Geometry: final body of the model. Coordinates: model frame, mm. A direction names the side the tool comes from. Give positions to 0.01 mm unless a question says otherwise; leave off trailing zeros. Write each loop counter-clockwise with the first axis right and the second up, starting at its lowest first coordinate (ties: lowest second). Pieces come first, ordered by that corner, then holes. Notation, with made-up numbers: M 57,0 L 66,0 A35 ccw 66,37 Z; hole C -10,12.25 d5. An arc over 180 degrees is marked long. Use one line per item in the form item = value. Start each with the question number.
Item 1: Section query A-A on z = 64. Return loops of the section in (x, y), then the cut area to 3 significant figures.
Item 2: Access query for faces 1 (the cylindrical face through (-1.08, -4.88, 51.33)), 2 (the cylindrical face through (4.57, 7.167, 1.972)). Directions: +Z, -Z, +X, -X, +Y, -Y. A direction counts if a zero-diameter tool reaches every point of the face in a straight line with its end or side. Return the directions, or none.
Item 3: Material intervals for line 1 along Y through (x, z) = (0, 40); line 2 along Z through (x, y) = (-1.25, -4.75); line 3 along Z through (x, y) = (6.5, 1.25), sorted ascending. Write a range as from..to.
Item 4: Contact query for flat-ended pins moving along their axis: P1, Ø6, axis at y = -6.5, z = 71.5, coming from the +X side; P2, Ø1.5, axis at y = -5, z = 51, coming from the -X side; P3, Ø4, axis at x = 0.5, z = 88.5, coming from the -Y side. Output: stop coordinate, or through.
from build123d import *

# Parameters (mm, degrees)
F0_R     = 8.5
F1_DEPTH = 4
F2_R     = 5
F3_DEPTH = 100
F8_R     = 0.5
F9_DEPTH = 114.1


with BuildPart() as f1:
    # F0 (on Top) → F1 (new body)
    with BuildSketch(Plane.XY):
        Circle(F0_R)
    extrude(amount=F1_DEPTH)

    # F2 (on Top) → F3 (join)
    with BuildSketch(Plane.XY):
        Circle(F2_R)
    extrude(amount=F3_DEPTH)

    # F4 (on Right) → F5 (revolve)
    with BuildSketch(Plane.YZ):
        with BuildLine():
            Line((3, 102), (0, 102))
            Line((0, 102), (0, 100))
            Line((0, 100), (5, 100))
            ThreePointArc((5, 100), (3.585786, 100.585786), (3, 102))
        make_face()
    revolve(axis=Axis((0, 0, 101), (0, 0, -1)))

    # F6 (on Right) → F7 (revolve)
    with BuildSketch(Plane.YZ):
        with BuildLine():
            Line((0, 104), (0, 102))
            Line((0, 102), (3, 102))
            ThreePointArc((3, 102), (2.414214, 103.414214), (1, 104))
            Line((1, 104), (0, 104))
        make_face()
    revolve(axis=Axis((0, 0, 103), (0, 0, 1)))

    # F8 (on face) → F9 (cut)
    with BuildSketch(Plane.XY.offset(104)):
        Circle(F8_R)
    extrude(amount=-F9_DEPTH, mode=Mode.SUBTRACT)


solid = f1.part
Answer sheet:
q1.outline = C 0,0 d10; hole C 0,0 d1
q1.area = 77.8 mm2
q2.face_1 = +Z
q2.face_2 = +Z, -Z
q3.line_1 = -5..-0.5, 0.5..5
q3.line_2 = 0..100
q3.line_3 = 0..4
q4.P1 = 3.57
q4.P2 = -2.63
q4.P3 = -5
